For this review, use the dimensioned drawing (mm, ordinates from the lowest corner) and the shaded views. Coordinates: 2 decimals unless noted, no trailing zeros. Loops run counter-clockwise (first coordinate to the right, second up) from the corner with the lowest first, then second, coordinate; pieces in that order, holes last. Notation, with made-up numbers: M -11,72.5 L 46,72.5 A8 cw 46,81.5 Z; hole C 89,6.5 d5. An arc over 180 degrees is marked long. Use CSV: the item, a comma, the result in double quotes. Start each with the question number.
1. Add section D-D, the plane z = 0.65. Write out the cut boundary in (x, y), then the cut area to 3 significant figures.
2. Add section C-C, the plane z = 2.4. Write out the cut boundary in (x, y), then the cut area to 3 significant figures.
3. Clearance check with flat-ended pins moving along their axes: P1, Ø3, axis at x = 15, y = 6, coming from the +Z side; P2, Ø1.4, axis at x = 5, y = 6, coming from the -Z side. State where each tip first meets the part, or that it passes through.
4. Add section A-A, the plane x = 15. Write out the cut boundary in (y, z).
5. For L1, parallel to X at y = 6, z = 1.1; L2, parallel to Y at x = 5, z = 1.45; L3, parallel to X at y = 5.5, z = 2.15, list the stretches that pass through material, from the lowest coordinate up.
6. Draft analysis for pull direction X (two halves, no side actions). For the marked faces 1, 2, 3 and 4, state which applies: +X half, -X half, draft (parallel to the pull), parting line (faces both ways), or undercut.
7. Add section B-B, the plane y = 6. Write out the cut boundary in (x, z).
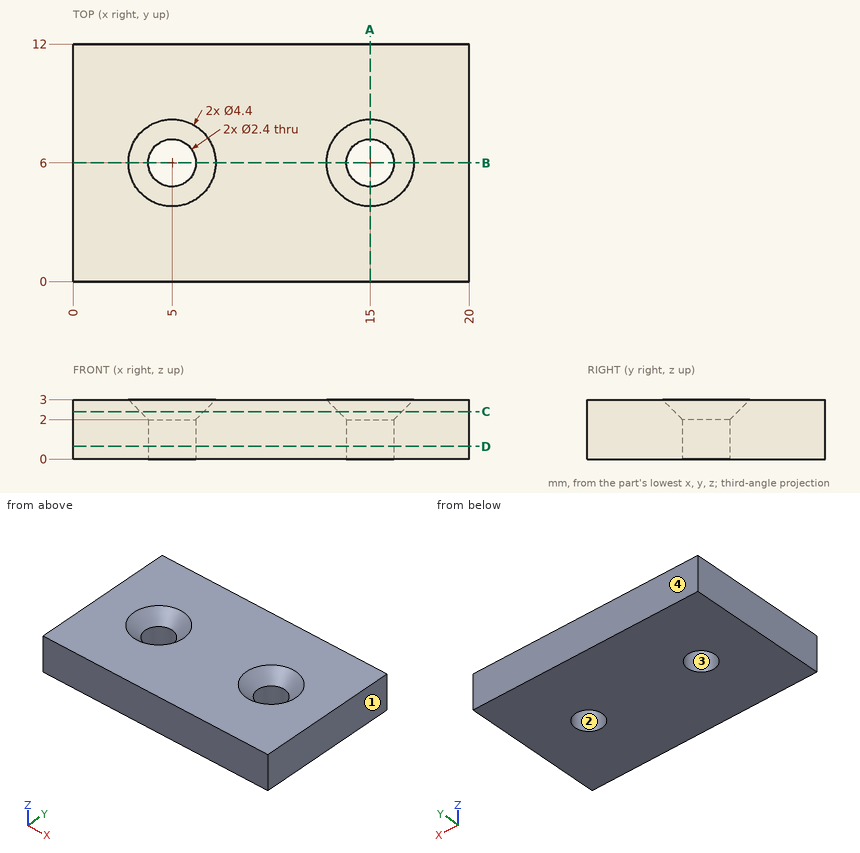
Computed:
1,outline,"M 0,0 L 20,0 L 20,12 L 0,12 Z; hole C 5,6 d2.4; hole C 15,6 d2.4"
1,area,"231 mm^2"
2,outline,"M 0,0 L 20,0 L 20,12 L 0,12 Z; hole C 5,6 d3.2; hole C 15,6 d3.2"
2,area,"224 mm^2"
3,P1,"stops at z = 2.3"
3,P2,"passes through"
4,outline,"M 0,0 L 4.8,0 L 4.8,2 L 3.8,3 L 0,3 Z; M 7.2,0 L 12,0 L 12,3 L 8.2,3 L 7.2,2 Z"
5,L1,"x = 0 to 3.8, 6.2 to 13.8, 16.2 to 20"
5,L2,"y = 0 to 4.8, 7.2 to 12"
5,L3,"x = 0 to 3.75, 6.25 to 13.75, 16.25 to 20"
6,face 1,"+X half"
6,face 2,"undercut"
6,face 3,"undercut"
6,face 4,"draft"
7,outline,"M 0,0 L 3.8,0 L 3.8,2 L 2.8,3 L 0,3 Z; M 6.2,0 L 13.8,0 L 13.8,2 L 12.8,3 L 7.2,3 L 6.2,2 Z; M 16.2,0 L 20,0 L 20,3 L 17.2,3 L 16.2,2 Z"
